Can you work these out from the model? Positions are in its coordinate system, mm. A direction names the side the tool comes from. Give positions to 0.01 mm unless a question says otherwise; leave off trailing zeros. Write each loop counter-clockwise with the first axis right and the second up, starting at its lowest first coordinate (ties: lowest second). Pieces come first, ordered by that corner, then holes. Notation, with made-up numbers: (-12, 52.5) - (17, 52.5) arc R14 cw to (17, 75.5) - close; hole circle Ø5 at (-31, 73.5). An arc over 180 degrees is marked (long way). Return JSON: item names as keys, results as strings. Group by question number.
Autodesk Inventor part; units mm, degrees
ref_plane "YZ Plane" through (0, 0, 0) normal (1, 0, 0) x (0, 1, 0)
ref_plane "XZ Plane" through (0, 0, 0) normal (0, 1, 0) x (-1, 0, 0)
ref_plane "XY Plane" through (0, 0, 0) normal (0, 0, 1) x (1, 0, 0)
sketch "Sketch1" plane through (0, 0, 0) normal (0, 0, 1) x (1, 0, 0)
  circle A0 centre (0, 0) radius 25.5
  dimension "d0" = 51
extrude "Extrusion1" add sketch "Sketch1" along normal blind 3
sketch "Sketch2" plane through (0, 0, 0) normal (0, 0, -1) x (-1, 0, 0)
  circle A0 centre (0, 0) radius 25.5
  circle A1 centre (0, 0) radius 14.5
  dimension "d3" = 29
extrude "Extrusion2" add sketch "Sketch2" along normal blind 90 contours A1
sketch "Sketch3" plane through (0, 0, 3) normal (0, 0, 1) x (1, 0, 0)
  circle A0 centre (0, 0) radius 25.5
  circle A1 centre (0, 0) radius 20.5
  circle A2 centre (0, 20.5) radius 1.5
  circle A3 centre (-14.4957, 14.4957) radius 1.5
  circle A4 centre (-20.5, 0) radius 1.5
  circle A5 centre (-14.4957, -14.4957) radius 1.5
  circle A6 centre (0, -20.5) radius 1.5
  circle A7 centre (14.4957, -14.4957) radius 1.5
  circle A8 centre (20.5, 0) radius 1.5
  circle A9 centre (14.4957, 14.4957) radius 1.5
  dimension "d6" = 41
  dimension "d7" = 3
  dimension "d10" = 360
extrude "Extrusion3" cut sketch "Sketch3" against normal through all contours A1 A8 | A1 A8 | A9 A1 | A1 A9 | A7 A1 | A1 A7 | A2 A1 | A1 A2 | A6 A1 | A1 A6 | A3 A1 | A1 A3 | A5 A1 | A1 A5 | A4 A1 | A1 A4
sketch "Sketch4" plane through (0, 0, 3) normal (0, 0, 1) x (1, 0, 0)
  circle A0 centre (0, 0) radius 25.5
  circle A1 centre (0, 0) radius 11
  dimension "d14" = 22
extrude "Extrusion4" cut sketch "Sketch4" against normal through all contours A1
sketch "Sketch5" plane through (0, 0, 0) normal (1, 0, 0) x (0, 1, 0)
  line L0 (0, -10.5) -> (0, -65.5)
  arc A0 (-7.5, -65.5) -> (7.5, -65.5) centre (0, -65.5) ccw
  arc A1 (7.5, -10.5) -> (-7.5, -10.5) centre (0, -10.5) ccw
  line L1 (7.5, -10.5) -> (7.5, -65.5)
  line L2 (-7.5, -65.5) -> (-7.5, -10.5)
  line L3 (25.5, 3) -> (-25.5, 3)
  point P0 (0, 0)
  point P1 (0, -3)
  point P2 (0, 3)
  dimension "d17" = 7.5
  dimension "d18" = 7.5
  dimension "d22" = 55
  dimension "d23" = 13.5
extrude "Extrusion5" cut sketch "Sketch5" along normal through all both and the other way through all
properties part number "11 CROSSHEAD GUIDE" material "Steel AISI 1020 107 HR"
1) We'd pull the mould along Z, two halves only. Please class faces 4 (the face through (11, -11, 0)), 5 (the face through (-10, 7.5, -38)), 6 (the face through (-5.5, 24.9, 1.5)), 7 (the face through (10, -7.5, -38)): pulls with the +Z half, pulls with the -Z half, needs draft (parallel to the pull), parting line crosses it, or undercut.
2) Imagine slicing it at C-C, the plane z = -39. Write out the boundary of the cut face in (x, y), and give its area (3 significant figures).
3) Imagine slicing it at D-D, the plane x = 20.5. Write out the boundary of the cut face in (y, z), and give its area (3 significant figures).
4) Will these pins go through, and if not, where does the flat tip stop? pin 1 Ø4 at (x, z) = (-11.5, -17) entering from +Y; pin 2 Ø10 at (x, y) = (-15, 3.5) entering from -Z; pin 3 Ø1.3 at (x, z) = (-10.5, -26) entering from +Y; pin 4 Ø1.3 at (x, z) = (11, -33) entering from -Y.
5) Imagine slicing it at A-A, the plane x = 0. Write out the boundary of the cut face in (y, z).
6) Imagine slicing it at B-B, the plane y = 0. Write out the boundary of the cut face in (x, z), and give its area (3 significant figures).
7) On a 3-axis mill with a long thin cutter (end or side, diameter ignored), from which of +Z, -Z, +X, -X, +Y, -Y can I reach the whole of each face in a straight line? I mean faces 1 (the face through (-10, -7.5, -38)), 2 (the face through (11.51, 8.82, -44.37)), 3 (the face through (15.93, -14.05, 1.52)). Say none if no direction works.
8) I need wall thicknesses on line 1 along Y through (x, z) = (0, -27); line 2 along Z through (x, y) = (1, 18); line 3 along Y through (x, z) = (20.5, 1.2). Which ranges of each line are inside material? Lowest first, please.
Resolved:
{
 "1": {"face 4": "pulls with the -Z half", "face 5": "undercut", "face 6": "needs draft", "face 7": "undercut"},
 "2": {"outline": "(-12.41, -7.5) arc R14.5 ccw to (12.41, -7.5) - (8.05, -7.5) arc R11 cw to (-8.05, -7.5) - close; (-12.41, 7.5) - (-8.05, 7.5) arc R11 cw to (8.05, 7.5) - (12.41, 7.5) arc R14.5 ccw to start", "area": "168 mm^2"},
 "3": {"outline": "(-15.17, 0) - (-1.5, 0) - (-1.5, 3) - (-15.17, 3) - close; (1.5, 0) - (15.17, 0) - (15.17, 3) - (1.5, 3) - close", "area": "82.0 mm^2"},
 "4": {"pin 1": "y = 10.95", "pin 2": "z = -90", "pin 3": "y = 10.64", "pin 4": "y = -10.16"},
 "5": {"outline": "(-25.5, 0) - (-22, 0) - (-22, 3) - (-25.5, 3) - close; (-19, 0) - (-14.5, 0) - (-14.5, -90) - (-11, -90) - (-11, 3) - (-19, 3) - close; (11, -90) - (14.5, -90) - (14.5, 0) - (19, 0) - (19, 3) - (11, 3) - close; (22, 0) - (25.5, 0) - (25.5, 3) - (22, 3) - close"},
 "6": {"outline": "(-25.5, 0) - (-22, 0) - (-22, 3) - (-25.5, 3) - close; (-19, 0) - (-14.5, 0) - (-14.5, -3) - (-11, -3) - (-11, 3) - (-19, 3) - close; (-14.5, -90) - (-11, -90) - (-11, -73) - (-14.5, -73) - close; (11, -90) - (14.5, -90) - (14.5, -73) - (11, -73) - close; (11, -3) - (14.5, -3) - (14.5, 0) - (19, 0) - (19, 3) - (11, 3) - close; (22, 0) - (25.5, 0) - (25.5, 3) - (22, 3) - close", "area": "209 mm^2"},
 "7": {"face 1": "+X, -X", "face 2": "-Z", "face 3": "+Z, -Z"},
 "8": {"line 1": "-14.5 to -11, 11 to 14.5", "line 2": "0 to 3", "line 3": "-15.17 to -1.5, 1.5 to 15.17"}
}
